```python
from build123d import *

# Parameters (mm, degrees)
SKETCH_1_W             = 200
SKETCH_1_H             = 200
EXTRUDE_1_DEPTH        = 3
SKETCH_5_W             = 200
SKETCH_5_H             = 200
EXTRUDE_2_DEPTH        = 3
SKETCH_2_R             = 2.55
SKETCH_2_R_2           = 2.15
CUT_EXTRUDE_1_DEPTH    = 10
CHAMFER_1_SIZE         = 10
HOLE_WIZARD_M4_1_D     = 4.5
HOLE_WIZARD_M4_1_DEPTH = 6
HOLE_WIZARD_M4_1_TIP   = 1.351936393


with BuildPart() as part:
    # 스케치1 → 보스-돌출1 (new body)
    with BuildSketch(Plane.XY):
        Rectangle(SKETCH_1_W, SKETCH_1_H)
    extrude(amount=EXTRUDE_1_DEPTH)

    # 스케치5 → 보스-돌출2 (add)
    with BuildSketch(Plane.XY.offset(3)):
        Rectangle(SKETCH_5_W, SKETCH_5_H)
    extrude(amount=EXTRUDE_2_DEPTH)

    # 스케치2 → 컷-돌출1 (cut)
    with BuildSketch(Plane.XY):
        with Locations((-36.5, 15)):
            Circle(SKETCH_2_R)
        with Locations((-36.5, -15)):
            Circle(SKETCH_2_R)
        with Locations((-6.5, 0)):
            Circle(SKETCH_2_R_2)
        with Locations((15, 36.5)):
            Circle(SKETCH_2_R)
        with Locations((-15, 36.5)):
            Circle(SKETCH_2_R)
        with Locations((0, 6.5)):
            Circle(SKETCH_2_R_2)
        with Locations((36.5, -15)):
            Circle(SKETCH_2_R)
        with Locations((36.5, 15)):
            Circle(SKETCH_2_R)
        with Locations((6.5, 0)):
            Circle(SKETCH_2_R_2)
        with Locations((-15, -36.5)):
            Circle(SKETCH_2_R)
        with Locations((15, -36.5)):
            Circle(SKETCH_2_R)
        with Locations((0, -6.5)):
            Circle(SKETCH_2_R_2)
    extrude(amount=CUT_EXTRUDE_1_DEPTH, mode=Mode.SUBTRACT)

    # 모따기1
    # the kernel refuses this chamfer: 10 mm, written as the material it takes off along each edge
    with BuildSketch(Plane(origin=(-125.71682988, 100, 0), x_dir=(0, 0.027495876610586317, 0.9996219169112968), z_dir=(1, 0, 0)), Plane(origin=(-100, -125.71682988, 0), x_dir=(-0.027495876610586317, 0, 0.9996219169112968), z_dir=(0, 1, 0)), Plane(origin=(100, 125.71682988, 0), x_dir=(0.027495876610586317, 0, 0.9996219169112968), z_dir=(0, -1, 0))) as chamfer_1_piece_1:
        Polygon((CHAMFER_1_SIZE * 0.999621916911, CHAMFER_1_SIZE * 0.0274958766106), (-CHAMFER_1_SIZE * 0.0274958766106, CHAMFER_1_SIZE * 0.999621916911), (0, 0), align=None)
    extrude(amount=251.433659759, mode=Mode.SUBTRACT)
    with BuildSketch(Plane(origin=(125.71682988, -100, 0), x_dir=(0, 0.9996219169112968, -0.027495876610586372), z_dir=(-1, 0, 0))) as chamfer_1_piece_2:
        Polygon((CHAMFER_1_SIZE * 0.999621916911, -CHAMFER_1_SIZE * 0.0274958766106), (-CHAMFER_1_SIZE * 0.0274958766106, -CHAMFER_1_SIZE * 0.999621916911), (0, 0), align=None)
    extrude(amount=251.433659759, mode=Mode.SUBTRACT)

    # M4 여유 구멍1
    with Locations(Plane.XY.offset(6)):
        with Locations((-86, -86), (-86, 86), (86, 86), (86, -86), (-86, -36), (-36, -86), (36, -86), (86, -36), (86, 36), (-36, 86), (36, 86), (-86, 36)):
            Hole(HOLE_WIZARD_M4_1_D / 2, depth=HOLE_WIZARD_M4_1_DEPTH)
            with Locations((0, 0, -(HOLE_WIZARD_M4_1_DEPTH + HOLE_WIZARD_M4_1_TIP / 2))):  # 118° drill point
                Cone(0, HOLE_WIZARD_M4_1_D / 2, HOLE_WIZARD_M4_1_TIP, mode=Mode.SUBTRACT)


solid = part.part
```
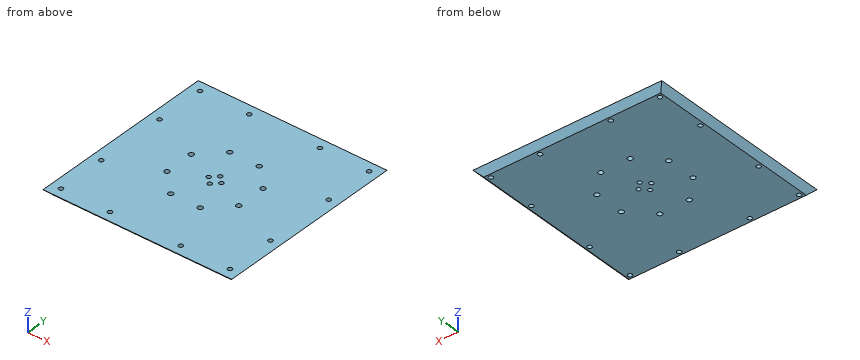
For this review, take the finished solid that the model builds, in its own axes (mm). Round coordinates to 2 decimals unless told otherwise and drop trailing zeros. Write each loop counter-clockwise with the first axis right and the second up, starting at its lowest first coordinate (ties: lowest second). Pieces come first, ordered by that corner, then holes. Notation, with made-up numbers: (-9, 5) - (49, 5) arc R16 cw to (49, 28) - close; hole circle Ø3 at (44, 51). An arc over 180 degrees is marked (long way). Use CSV: the item, a comma, the result in double quotes.
1) Wall thickness on line 1 along Y through (x, z) = (36.5, 2.7); line 2 along Y through (x, z) = (36, 2.5); line 3 along Y through (x, z) = (-16, 1.75): over which ranges is each line inside the solid? List them lowest first. Write a range as from..to.
Conclusion:
line 1,"y = -92.7..-88.19, -83.81..-17.55, -12.45..12.45, 17.55..83.81, 88.19..92.7"
line 2,"y = -92.5..-88.25, -83.75..-17.5, -12.5..12.5, 17.5..83.75, 88.25..92.5"
line 3,"y = -91.75..-38.85, -34.15..34.15, 38.85..91.75"
2) Add section D-D on x = 54. Write out the cut boundary in (y, z), and give its area (3 significant figures).
Conclusion:
outline,"(-96, 6) - (-90, 0) - (90, 0) - (96, 6) - close"
area,"1,120 mm^2"
3) Add section A-A on y = -15. Write out the cut boundary in (x, z).
Conclusion:
outline,"(-96, 6) - (-90, 0) - (-39.05, 0) - (-39.05, 6) - close; (-33.95, 0) - (33.95, 0) - (33.95, 6) - (-33.95, 6) - close; (39.05, 0) - (90, 0) - (96, 6) - (39.05, 6) - close"
4) Clearance check with a flat-ended pin moving along its axis: pin 1 Ø3.5 at (x, y) = (-36, -86) entering from +Z. State where the tip first meets the part, or that it passes through.
Conclusion:
pin 1,"passes through"
5) Add section C-C on y = -86. Write out the cut boundary in (x, z).
Conclusion:
outline,"(-96, 6) - (-90, 0) - (-88.25, 0) - (-88.25, 6) - close; (-83.75, 0) - (-38.25, 0) - (-38.25, 6) - (-83.75, 6) - close; (-33.75, 0) - (33.75, 0) - (33.75, 6) - (-33.75, 6) - close; (38.25, 0) - (83.75, 0) - (83.75, 6) - (38.25, 6) - close; (88.25, 0) - (90, 0) - (96, 6) - (88.25, 6) - close"
6) Add section B-B on z = 3. Count the separate pieces of the cut face and the enclosed holes in it, and give its area (3 significant figures).
Conclusion:
separate pieces,"1"
enclosed holes,"24"
area,"34,200 mm^2"
